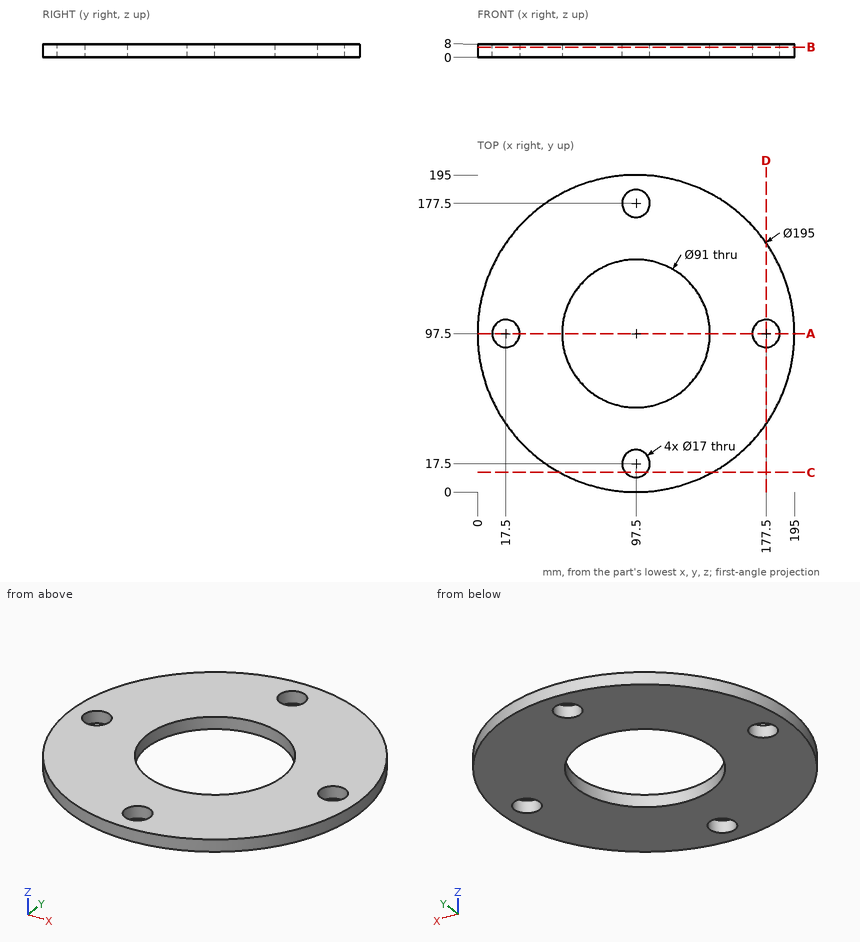
Job drawing, mm, ordinate dimensions from the low corner. One solid piece. Round coordinates to 2 decimals unless told otherwise and drop trailing zeros. Loops run counter-clockwise (first coordinate to the right, second up) from the corner with the lowest first, then second, coordinate; pieces in that order, holes last.
Item 1: Drop a flat-ended pin along its axis: P1, Ø1, axis at x = 125.5, z = 3.5, coming from the +Y side. Give the stop position or say it passes through.
Item 2: Drill centre lines: line 1 (X direction, y = 86, z = 1); line 2 (X direction, y = 173, z = 3.5); line 3 (Y direction, x = 128.5, z = 6.75). Where is each one in solid material? Low to high.
Item 3: Cut at D-D, the plane x = 177.5. Give the cut face in (y, z), then the cut area to 3 significant figures.
Item 4: Cut at B-B, the plane z = 6. Give the cut face in (x, y), then the cut area to 3 significant figures.
Item 5: Cut at A-A, the plane y = 97.5. Give the cut face in (x, z).
Item 6: Cut at C-C, the plane y = 12. Give the cut face in (x, z), then the cut area to 3 significant figures.
A:
1. P1: stops at y = 191.04
2. line 1: x = 0.68 to 53.48, 141.52 to 194.32
2. line 2: x = 35.81 to 90.29, 104.71 to 159.19
2. line 3: y = 5.06 to 64.19, 130.81 to 189.94
3. outline: (41.77, 0) - (89, 0) - (89, 8) - (41.77, 8) - close; (106, 0) - (153.23, 0) - (153.23, 8) - (106, 8) - close
3. area: 756 mm2
4. outline: circle Ø195 at (97.5, 97.5); hole circle Ø17 at (17.5, 97.5); hole circle Ø91 at (97.5, 97.5); hole circle Ø17 at (97.5, 17.5); hole circle Ø17 at (97.5, 177.5); hole circle Ø17 at (177.5, 97.5)
4. area: 22,500 mm2
5. outline: (0, 0) - (9, 0) - (9, 8) - (0, 8) - close; (26, 0) - (52, 0) - (52, 8) - (26, 8) - close; (143, 0) - (169, 0) - (169, 8) - (143, 8) - close; (186, 0) - (195, 0) - (195, 8) - (186, 8) - close
6. outline: (50.64, 0) - (91.02, 0) - (91.02, 8) - (50.64, 8) - close; (103.98, 0) - (144.36, 0) - (144.36, 8) - (103.98, 8) - close
6. area: 646 mm2
